```python
from build123d import *

# Parameters (mm, degrees)
CHAMFER1_SIZE       = 0.05
BOSS_EXTRUDE1_START = -2
SKETCH4_R           = 1.5
BOSS_EXTRUDE1_DEPTH = 2
SKETCH5_OUTSIDE_W   = 20.904
SKETCH5_OUTSIDE_H   = 19.856
SKETCH5_OUTSIDE_R   = 3.478175124
CUT_EXTRUDE2_DEPTH  = 2
CUT_EXTRUDE2_DRAFT  = -60
SKETCH6_OUTSIDE_W   = 20.904
SKETCH6_OUTSIDE_H   = 19.856
SKETCH6_OUTSIDE_R   = 3.478175124
CUT_EXTRUDE3_DEPTH  = 2
CUT_EXTRUDE3_DRAFT  = -60
FILLET1_R           = 0.075


with BuildPart() as part:
    # Sketch1 → Revolve1 (revolve)
    with BuildSketch(Plane.XY):
        with BuildLine():
            Line((0, 16.598076211), (0, 0))
            Line((0, 0), (1.5, 0))
            Line((1.5, 0), (1.5, 11))
            ThreePointArc((1.5, 11), (2.897777479, 14.374533347), (0, 16.598076211))
        make_face()
    revolve(axis=Axis((0, 16.598076211, 0), (0, -1, 0)))

    # Chamfer1
    chamfer1_edges = [part.edges().sort_by_distance(p)[0] for p in [
        (-1.5, 0, 0),
    ]]
    chamfer(chamfer1_edges, length=CHAMFER1_SIZE)

    # Sketch4 → Boss-Extrude1 (add)
    with BuildSketch(Plane(origin=(0, 7, 0), x_dir=(-1, 0, 0), z_dir=(0, -1, 0)).offset(BOSS_EXTRUDE1_START)):
        Polygon((1.983846765, -3.492079839), (4.016153235, -0.027978224), (2.032306471, 3.464101615), (-1.983846765, 3.492079839), (-4.016153235, 0.027978224), (-2.032306471, -3.464101615), align=None)
        with Locations(Location((0, 0, 0), (0, 0, 270))):
            Circle(SKETCH4_R, mode=Mode.SUBTRACT)
    extrude(amount=BOSS_EXTRUDE1_DEPTH)


with BuildPart() as cut_extrude2_tool:
    # Sketch5 outside → Cut-Extrude2 (with draft: the straight prism first)
    with BuildSketch(Plane.XZ.offset(-7)):
        Rectangle(SKETCH5_OUTSIDE_W, SKETCH5_OUTSIDE_H)
        Circle(SKETCH5_OUTSIDE_R, mode=Mode.SUBTRACT)
    extrude(amount=-CUT_EXTRUDE2_DEPTH)
    # Cut-Extrude2: the draft: its side faces are tilted about the plane it starts from
    cut_extrude2_sides = [cut_extrude2_tool.faces().sort_by_distance(p)[0] for p in [
        (0, 8, -9.928),
        (10.452, 8, 0),
        (0, 8, 9.928),
        (-10.452, 8, 0),
        (-3.478175124, 8, 0),
    ]]
    draft(cut_extrude2_sides, Plane.XZ.offset(-7), CUT_EXTRUDE2_DRAFT)


with BuildPart() as part_1:
    add(part.part)

    # Cut-Extrude2: cut by cut_extrude2_tool
    add(cut_extrude2_tool.part, mode=Mode.SUBTRACT)


with BuildPart() as cut_extrude3_tool:
    # Sketch6 outside → Cut-Extrude3 (with draft: the straight prism first)
    with BuildSketch(Plane(origin=(0, 9, 0), x_dir=(1, 0, 0), z_dir=(0, 1, 0))):
        Rectangle(SKETCH6_OUTSIDE_W, SKETCH6_OUTSIDE_H)
        Circle(SKETCH6_OUTSIDE_R, mode=Mode.SUBTRACT)
    extrude(amount=-CUT_EXTRUDE3_DEPTH)
    # Cut-Extrude3: the draft: its side faces are tilted about the plane it starts from
    cut_extrude3_sides = [cut_extrude3_tool.faces().sort_by_distance(p)[0] for p in [
        (0, 8, 9.928),
        (10.452, 8, 0),
        (0, 8, -9.928),
        (-10.452, 8, 0),
        (-3.478175124, 8, 0),
    ]]
    draft(cut_extrude3_sides, Plane(origin=(0, 9, 0), x_dir=(1, 0, 0), z_dir=(0, 1, 0)), CUT_EXTRUDE3_DRAFT)


with BuildPart() as part_2:
    add(part_1.part)

    # Cut-Extrude3: cut by cut_extrude3_tool
    add(cut_extrude3_tool.part, mode=Mode.SUBTRACT)

    # Fillet1
    fillet1_edges = [part_2.edges().sort_by_distance(p)[0] for p in [
        (-1.5, 11, 0),
    ]]
    fillet(fillet1_edges, radius=FILLET1_R)


solid = part_2.part
```
Here's how the part is built. I have some questions about the finished solid (model axes, mm). A direction names the side the tool comes from. Coordinates: 2 decimals unless noted, no trailing zeros. Order: outer loops, then holes, each group sorted by start corner. A loop starts at its lowest first (then second) coordinate and runs counter-clockwise, first axis right, second up.
Item 1: I'm going to push flat-ended pins straight in: pin 1 Ø1 at (y, z) = (4.5, 0.5) entering from -X; pin 2 Ø1.5 at (y, z) = (1.5, 1.5) entering from +X; pin 3 Ø1 at (x, z) = (3, -0.5) entering from +Y. Where does each tip first touch, or does it pass through?
Response values:
pin 1: stops at x = -1.5
pin 2: stops at x = 1.3
pin 3: stops at y = 15.19
Item 2: I need wall thicknesses on probe 1 along Z at (x, y) = (0, 10.75); probe 2 along Y at (x, z) = (-1.75, -2.5); probe 3 along Z at (x, y) = (-0.5, 7.5). Which ranges of each line are inside material? Lowest first, please.
Response values:
probe 1: z = -1.5 to 1.5
probe 2: y = 7 to 9
probe 3: z = -3.47 to 3.48
Item 3: Which directions (+Z, -Z, +X, -X, +Y, -Y) give clear straight access to the entire face, cutting with the end or side of a thin tool? Please do faces 1 (the face through (1.43, 3.57, 0.45)), 2 (the face through (-3.67, 7.11, 0.03)), 3 (the face through (1.43, 9.99, 0.45)).
Response values:
face 1: -Y
face 2: -X, -Y
face 3: none
Item 4: If we section it at A-A, the plane y = 1.5: List the corners of the cut face in (x, z) for me, then the cut area to 3 significant figures.
Response values:
outline: circle Ø3 at (0, 0)
area: 7.07 mm2
Item 5: Thinking about a two-plate mould opening in Y: for faces 4 (the face through (3.67, 7.11, -0.03)), 5 (the face through (-0.7, 9, 1.5)), 6 (the face through (-1.819, 8.891, 3.183)), which applies, pulls with the +Y half, pulls with the -Y half, needs draft (parallel to the pull), parting line crosses it, or undercut?
Response values:
face 4: pulls with the -Y half
face 5: undercut
face 6: pulls with the +Y half
